Autodesk Inventor part; units mm, degrees
ref_plane "YZ Plane" through (0, 0, 0) normal (1, 0, 0) x (0, 1, 0)
ref_plane "XZ Plane" through (0, 0, 0) normal (0, 1, 0) x (-1, 0, 0)
ref_plane "XY Plane" through (0, 0, 0) normal (0, 0, 1) x (1, 0, 0)
sketch "Sketch1" plane through (0, 0, 0) normal (0, 0, 1) x (1, 0, 0)
  line L0 (-42.8727, 26.6374) -> (-4.7727, 26.6374)
  line L1 (-4.7727, 26.6374) -> (-4.7727, -11.4626)
  line L2 (-4.7727, -11.4626) -> (-42.8727, -11.4626)
  line L3 (-42.8727, -11.4626) -> (-42.8727, 26.6374)
  point P0 (0, 0)
  dimension "d0" = 38.1
  dimension "d1" = 38.1
extrude "Extrusion1" add sketch "Sketch1" along normal blind 6
sketch "Sketch2" plane through (0, 0, 6) normal (0, 0, 1) x (1, 0, 0)
  line L0 (-41.7124, 24.7081) -> (-6.0889, 24.7081)
  line L1 (-6.0889, 24.7081) -> (-6.0889, -9.5927)
  line L2 (-6.0889, -9.5927) -> (-41.7124, -9.5927)
  line L3 (-41.7124, -9.5927) -> (-41.7124, 24.7081)
  point P0 (0, 0)
extrude "Extrusion2" add sketch "Sketch2" along normal blind 8
sketch "Sketch3" plane through (0, 0, 14) normal (0, 0, 1) x (1, 0, 0)
  line L0 (-4.7727, 26.6374) -> (-42.8727, 26.6374)
  line L1 (-4.7727, -11.4626) -> (-4.7727, 26.6374)
  line L2 (-42.8727, 26.6374) -> (-4.7727, 26.6374)
  line L3 (-4.7727, 26.6374) -> (-4.7727, -11.4626)
  line L4 (-4.7727, -11.4626) -> (-42.8727, -11.4626)
  line L5 (-42.8727, -11.4626) -> (-42.8727, 26.6374)
  point P0 (0, 0)
extrude "Extrusion3" add sketch "Sketch3" along normal blind 6
sketch "Sketch4" plane through (0, 0, 20) normal (0, 0, 1) x (1, 0, 0)
  circle A0 centre (-23.8227, 7.5874) radius 5
  line L0 (-4.7727, 26.6374) -> (-42.8727, 26.6374)
  line L1 (-4.7727, -11.4626) -> (-4.7727, 26.6374)
  point P0 (0, 0)
  dimension "d8" = 10
  dimension "d9" = 19.05
  dimension "d10" = 19.05
extrude "Extrusion4" add sketch "Sketch4" along normal blind 7
properties part number "rev motor"
Geometry check sheet. Reference: the model listing, model coordinates, mm. A direction names the side the tool comes from. Coordinates: 2 decimals unless noted, no trailing zeros. Order: outer loops, then holes, each group sorted by start corner. A loop starts at its lowest first (then second) coordinate and runs counter-clockwise, first axis right, second up. Notation, with made-up numbers: (34.5, -18) - (65.5, -18) arc R21 cw to (65.5, 2) - close; hole circle Ø10 at (2, 12). An arc over 180 degrees is marked (long way). Use one line per item in the form item = value.
1. Access from +Z, -Z, +X, -X, +Y, -Y to the whole of each face (thin tool, end or side, straight path). Record for faces 1 (the face through (-24, -9.593, 10)), 2 (the face through (-24, 24.708, 10)), 3 (the face through (-6.089, 8, 10)).
Here are the results:
face_1 = +X, -X, -Y
face_2 = +X, -X, +Y
face_3 = +X, +Y, -Y
2. Section check C-C (z = 7.5). Record the boundary of the cut face in (x, y), then the cut area to 3 significant figures.
Here are the results:
outline = (-41.71, -9.59) - (-6.09, -9.59) - (-6.09, 24.71) - (-41.71, 24.71) - close
area = 1,220 mm²
3. Section check B-B (y = 18). Record the boundary of the cut face in (x, z), then the cut area to 3 significant figures.
Here are the results:
outline = (-42.87, 0) - (-4.77, 0) - (-4.77, 6) - (-6.09, 6) - (-6.09, 14) - (-4.77, 14) - (-4.77, 20) - (-42.87, 20) - (-42.87, 14) - (-41.71, 14) - (-41.71, 6) - (-42.87, 6) - close
area = 742 mm²
4. Draft check along Z on faces 4 (the face through (-28, 12, 20)), 5 (the face through (-24, 26.637, 3)), 6 (the face through (-25, -11, 6)), 7 (the face through (-25, -11, 14)). Enter one of: pulls with the +Z half, pulls with the -Z half, needs draft (parallel to the pull), parting line crosses it, or undercut.
Here are the results:
face_4 = pulls with the +Z half
face_5 = needs draft
face_6 = undercut
face_7 = undercut
5. Scan lines: line 1 (Z direction, x = -27, y = 25.5); line 2 (Z direction, x = -23, y = 21.5); line 3 (X direction, y = -1.5, z = 13). Record each from-to range of solid material in increasing order.
Here are the results:
line_1 = 0 to 6, 14 to 20
line_2 = 0 to 20
line_3 = -41.71 to -6.09
6. Section check D-D (z = 22). Record the boundary of the cut face in (x, y), then the cut area to 3 significant figures.
Here are the results:
outline = circle Ø10 at (-23.82, 7.59)
area = 78.5 mm²
7. Gauge pin test, flat ends, axial feed: pin 1 (2.5 mm diameter, centred on y = 2, z = 8.5, fed in from +X); pin 2 (6.5 mm diameter, centred on x = -21, z = 10.5, fed in from -Y); pin 3 (2.5 mm diameter, centred on x = -28.5, z = 9.5, fed in from +Y). Record the tip position at first contact, or that the pin passes through.
Here are the results:
pin_1 = -6.09
pin_2 = -9.59
pin_3 = 24.71
8. Section check A-A (x = -14.5). Record the boundary of the cut face in (y, z).
Here are the results:
outline = (-11.46, 0) - (26.64, 0) - (26.64, 6) - (24.71, 6) - (24.71, 14) - (26.64, 14) - (26.64, 20) - (-11.46, 20) - (-11.46, 14) - (-9.59, 14) - (-9.59, 6) - (-11.46, 6) - close
